Check sheet for the modelled part. Datum: model origin and axes. Units: mm. Give positions to 0.01 mm unless a question says otherwise; leave off trailing zeros. Order: outer loops, then holes, each group sorted by start corner. A loop starts at its lowest first (then second) coordinate and runs counter-clockwise, first axis right, second up. Notation, with made-up numbers: (39.25, -22) -> (61.25, -22) arc R37 ccw to (61.25, 16) -> close; hole circle Ø2 at (58.25, -6.5). An arc over 180 degrees is marked (long way). One line per question, with ' | ' between items. Start each with the question number.
from build123d import *

# Parameters (mm, degrees)
SKETCH1_R           = 1.75
BOSS_EXTRUDE1_DEPTH = 2
CHAMFER1_SIZE       = 0.4


with BuildPart() as part:
    # Sketch1 → Boss-Extrude1 (new body)
    with BuildSketch(Plane(origin=(0, 0, 0), x_dir=(1, 0, 0), z_dir=(0, 1, 0))):
        Polygon((-32.6, 0), (32.6, 0), (32.6, 60.6), (23.8, 60.6), (23.8, 10), (-23.8, 10), (-23.8, 60.6), (-32.6, 60.6), align=None)
        with Locations(Location((-15, 5, 0), (0, 0, 270))):
            Circle(SKETCH1_R, mode=Mode.SUBTRACT)
        with Locations(Location((15, 5, 0), (0, 0, 270))):
            Circle(SKETCH1_R, mode=Mode.SUBTRACT)
    extrude(amount=BOSS_EXTRUDE1_DEPTH)

    # Chamfer1
    chamfer1_edges = [part.edges().sort_by_distance(p)[0] for p in [
        (28.2, 0, -60.6),
        (32.6, 0, -30.3),
        (0, 0, 0),
        (-32.6, 0, -30.3),
        (32.6, 2, -30.3),
        (28.2, 2, -60.6),
        (23.8, 2, -35.3),
        (-15, 0, -6.75),
        (-15, 2, -6.75),
        (0, 2, -10),
        (15, 0, -6.75),
        (15, 2, -6.75),
        (-23.8, 2, -35.3),
        (-28.2, 2, -60.6),
        (-32.6, 2, -30.3),
        (-28.2, 0, -60.6),
        (0, 2, 0),
        (-23.8, 0, -35.3),
        (0, 0, -10),
        (23.8, 0, -35.3),
    ]]
    chamfer(chamfer1_edges, length=CHAMFER1_SIZE)


solid = part.part
1. Scan lines: probe 1 along X at (y, z) = (1, -5); probe 2 along X at (y, z) = (1.2, -17); probe 3 along Z at (x, y) = (10, 1.1). Record each from-to range of solid material in increasing order.
2. Cross-section at D-D on z = -5. Record the boundary of the cut face in (x, y), and give its area (3 significant figures).
3. Mould release check, pull along X, two halves, no side actions. Record for faces 1 (the face through (16.735, 0.992, -5.228)), 2 (the face through (-3, 2, -8)): +X half, -X half, draft (parallel to the pull), parting line (faces both ways), or undercut.
4. Cross-section at A-A on x = 15. Record the boundary of the cut face in (y, z).
5. Go/stop test with flat-tipped pins: pin 1 (4.5 mm diameter, centred on x = 15, z = -5, fed in from -Y); pin 2 (4 mm diameter, centred on x = -15, z = -5, fed in from -Y); pin 3 (1 mm diameter, centred on x = 1.5, y = 1, fed in from -Z). Record where each tip stops, or that it passes through.
6. Cross-section at B-B on z = -37.5. Record the boundary of the cut face in (x, y), and give its area (3 significant figures).
7. Cross-section at C-C on y = 0.8. Record the boundary of the cut face in (x, z), and give its area (3 significant figures).
Response values:
1) probe 1: x = -32.6 to -16.75, -13.25 to 13.25, 16.75 to 32.6 | probe 2: x = -32.6 to -23.8, 23.8 to 32.6 | probe 3: z = -10 to 0
2) outline: (-32.6, 0.4) -> (-32.2, 0) -> (-17.15, 0) -> (-16.75, 0.4) -> (-16.75, 1.6) -> (-17.15, 2) -> (-32.2, 2) -> (-32.6, 1.6) -> close; (-13.25, 0.4) -> (-12.85, 0) -> (12.85, 0) -> (13.25, 0.4) -> (13.25, 1.6) -> (12.85, 2) -> (-12.85, 2) -> (-13.25, 1.6) -> close; (16.75, 0.4) -> (17.15, 0) -> (32.2, 0) -> (32.6, 0.4) -> (32.6, 1.6) -> (32.2, 2) -> (17.15, 2) -> (16.75, 1.6) -> close | area: 115 mm²
3) face 1: undercut | face 2: draft
4) outline: (0, -9.6) -> (0.4, -10) -> (1.6, -10) -> (2, -9.6) -> (2, -7.15) -> (1.6, -6.75) -> (0.4, -6.75) -> (0, -7.15) -> close; (0, -2.85) -> (0.4, -3.25) -> (1.6, -3.25) -> (2, -2.85) -> (2, -0.4) -> (1.6, 0) -> (0.4, 0) -> (0, -0.4) -> close
5) pin 1: stops at y = 0 | pin 2: stops at y = 0.15 | pin 3: stops at z = -10
6) outline: (-32.6, 0.4) -> (-32.2, 0) -> (-24.2, 0) -> (-23.8, 0.4) -> (-23.8, 1.6) -> (-24.2, 2) -> (-32.2, 2) -> (-32.6, 1.6) -> close; (23.8, 0.4) -> (24.2, 0) -> (32.2, 0) -> (32.6, 0.4) -> (32.6, 1.6) -> (32.2, 2) -> (24.2, 2) -> (23.8, 1.6) -> close | area: 34.6 mm²
7) outline: (-32.6, -60.6) -> (-23.8, -60.6) -> (-23.8, -10) -> (23.8, -10) -> (23.8, -60.6) -> (32.6, -60.6) -> (32.6, 0) -> (-32.6, 0) -> close; hole circle Ø3.5 at (-15, -5); hole circle Ø3.5 at (15, -5) | area: 1,520 mm²
